Autodesk Inventor part; units mm, degrees
ref_plane "YZ Plane" through (0, 0, 0) normal (1, 0, 0) x (0, 1, 0)
ref_plane "XZ Plane" through (0, 0, 0) normal (0, 1, 0) x (-1, 0, 0)
ref_plane "XY Plane" through (0, 0, 0) normal (0, 0, 1) x (1, 0, 0)
sketch "スケッチ1" plane through (0, 0, 0) normal (0, 0, 1) x (1, 0, 0)
  circle A0 centre (0, 0) radius 2
  dimension "d0" = 4
extrude "押し出し1" add sketch "スケッチ1" along normal blind 10
sketch "スケッチ2" plane through (0, 0, 0) normal (0, 0, -1) x (-1, 0, 0)
  circle A0 centre (0, 0) radius 4
  dimension "d3" = 8
extrude "押し出し2" add sketch "スケッチ2" along normal blind 1.5
thread "ねじ1"
chamfer "面取り1" distance 0.5 angle 30 1 edges at (4, 0, -1.5) measured on face at (-0.7574, 1.0973, -1.5)
properties part number "ネジローヘッドm4,10" material "鋼、高強度、低合金"
Input: part model. Units: mm. Frame: model coordinates. A direction names the side the tool comes from. Coordinates: 2 decimals unless noted, no trailing zeros. Write each loop counter-clockwise with the first axis right and the second up, starting at its lowest first coordinate (ties: lowest second). Pieces come first, ordered by that corner, then holes.
1) Pin query (flat end, axial travel): pin 1 Ø4 at (y, z) = (-2.5, 4.5) entering from +X; pin 2 Ø2 at (y, z) = (2, 4.5) entering from +X; pin 3 Ø1 at (x, y) = (2, -2.5) entering from +Z. Return the tip coordinate at first contact, or that it passes through.
2) Section C-C on z = 3.25. Output: boundary loops of the cut face in (x, y), and give its area (3 significant figures).
3) Section A-A on x = 0. Output: boundary loops of the cut face in (y, z), and give its area (3 significant figures).
4) Set-up query: faces 1 (the cylindrical face through (0, 2, 5)), 2 (the cylindrical face through (0.867, 3.905, -0.597)). Return all of +Z, -Z, +X, -X, +Y, -Y with unobstructed straight access to the full face (end or side cutting, diameter ignored); none if empty.
5) Material intervals for line 1 along Z through (x, y) = (1, 2); line 2 along Y through (x, z) = (0, 3.75); line 3 along X through (y, z) = (2.25, -0.25), sorted ascending.
Check result:
1. pin 1: stops at x = 1.94
1. pin 2: stops at x = 1.73
1. pin 3: stops at z = 0
2. outline: circle Ø4 at (0, 0)
2. area: 12.6 mm2
3. outline: (-4, -1.21) - (-3.5, -1.5) - (3.5, -1.5) - (4, -1.21) - (4, 0) - (2, 0) - (2, 10) - (-2, 10) - (-2, 0) - (-4, 0) - close
3. area: 51.9 mm2
4. face 1: +Z
4. face 2: +Z, -Z
5. line 1: z = -1.5 to 0
5. line 2: y = -2 to 2
5. line 3: x = -3.31 to 3.31
